Can you work these out from the model? Positions are in its coordinate system, mm. A direction names the side the tool comes from. Coordinates: 2 decimals unless noted, no trailing zeros. Write each loop counter-clockwise with the first axis right and the second up, starting at its lowest first coordinate (ties: lowest second). Pieces come first, ordered by that corner, then holes. Notation, with made-up numbers: M -22.75,-16.75 L 15.25,-16.75 A20 ccw 15.25,-7.75 Z; hole C 70.5,31 d10. An arc over 180 degrees is marked long. Answer as a JSON object with one key per item and string values. Group by question number.
from build123d import *

# Parameters (mm, degrees)
BOSS_EXTRUDE1_DEPTH = 1.4
BOSS_EXTRUDE2_START = -8.5
FRONT_FACE_3_W      = 155.03
FRONT_FACE_3_H      = 88.87
BOSS_EXTRUDE2_DEPTH = 8.5


with BuildPart() as part:
    # Front Face → Boss-Extrude1 (new body)
    with BuildSketch(Plane(origin=(0, 0, 0), x_dir=(1, 0, 0), z_dir=(0, 1, 0))):
        with BuildLine():
            ThreePointArc((0, 120.76), (2.928932188, 127.831067812), (10, 130.76))
            Line((10, 130.76), (202.96, 130.76))
            ThreePointArc((202.96, 130.76), (210.031067812, 127.831067812), (212.96, 120.76))
            Line((212.96, 120.76), (212.96, 10))
            ThreePointArc((212.96, 10), (210.031067812, 2.928932188), (202.96, 0))
            Line((202.96, 0), (10, 0))
            ThreePointArc((10, 0), (2.928932188, 2.928932188), (0, 10))
            Line((0, 10), (0, 120.76))
        make_face()
        with BuildLine():
            Line((10, 16), (10, 114.76))
            ThreePointArc((10, 114.76), (11.757359313, 119.002640687), (16, 120.76))
            Line((16, 120.76), (196.96, 120.76))
            ThreePointArc((196.96, 120.76), (201.202640687, 119.002640687), (202.96, 114.76))
            Line((202.96, 114.76), (202.96, 16))
            ThreePointArc((202.96, 16), (201.202640687, 11.757359313), (196.96, 10))
            Line((196.96, 10), (16, 10))
            ThreePointArc((16, 10), (11.757359313, 11.757359313), (10, 16))
        make_face(mode=Mode.SUBTRACT)
    extrude(amount=BOSS_EXTRUDE1_DEPTH)

    # Front Face_3 → Boss-Extrude2 (add)
    with BuildSketch(Plane(origin=(0, 0, 0), x_dir=(1, 0, 0), z_dir=(0, 1, 0)).offset(BOSS_EXTRUDE2_START)):
        with BuildLine():
            ThreePointArc((0, 10), (2.928932188, 2.928932188), (10, 0))
            Line((10, 0), (202.96, 0))
            ThreePointArc((202.96, 0), (210.031067812, 2.928932188), (212.96, 10))
            Line((212.96, 10), (212.96, 120.76))
            ThreePointArc((212.96, 120.76), (210.031067812, 127.831067812), (202.96, 130.76))
            Line((202.96, 130.76), (10, 130.76))
            ThreePointArc((10, 130.76), (2.928932188, 127.831067812), (0, 120.76))
            Line((0, 120.76), (0, 10))
        make_face()
        with Locations((106.48, 64.38)):
            Rectangle(FRONT_FACE_3_W, FRONT_FACE_3_H, mode=Mode.SUBTRACT)
    extrude(amount=BOSS_EXTRUDE2_DEPTH)


solid = part.part
Q1. Please list where these lines run through material, in increasing order: L1, parallel to Z at x = 165, y = -6.75 (3 decimals); L2, parallel to X at y = -7.5, z = -87 (3 decimals); L3, parallel to Y at x = 11.5, z = -71.5.
Q2. If we section it at C-C on x = 115: List the corners of the cut face in (y, z) for me (3 decimals).
Q3. Will this pin go through, and if not, where does the flat tip stop? pin 1 (1 mm diameter, centred on x = 186.5, z = -21, fed in from +Y).
Q4. On a 3-axis mill with a long thin cutter (end or side, diameter ignored), from which of +Z, -Z, +X, -X, +Y, -Y can I reach the whole of each face in a straight line? I mean faces 1 (the cylindrical face through (201.156, 0.69, -119.049)), 2 (the flat face through (183.995, -4, -64)), 3 (the flat face through (108, -4, -130.76)). Say none if no direction works.
Q5. If we section it at D-D on x = 188: List the corners of the cut face in (y, z) for me.
Q6. We'd pull the mould along X, two halves only. Please class faces 4 (the cylindrical face through (201.249, 0.69, -11.804)), 5 (the cylindrical face through (210.11, -3.62, -127.75)), 6 (the cylindrical face through (3, -3.6, -127.9)): pulls with the +X half, pulls with the -X half, needs draft (parallel to the pull), parting line crosses it, or undercut.
Q7. If we section it at A-A on z = -74.5: List the corners of the cut face in (x, y) for me (3 decimals).
Q8. If we section it at B-B on y = -2.5: List the corners of the cut face in (x, z) for me (3 decimals), and give its area (3 significant figures).
Reply:
{
 "1": {"L1": "-130.76 to -108.815, -19.945 to 0", "L2": "0 to 28.965, 183.995 to 212.96", "L3": "-8.5 to 0"},
 "2": {"outline": "M -8.5,-130.76 L 1.4,-130.76 L 1.4,-120.76 L 0,-120.76 L 0,-108.815 L -8.5,-108.815 Z; M -8.5,-19.945 L 0,-19.945 L 0,-10 L 1.4,-10 L 1.4,0 L -8.5,0 Z"},
 "3": {"pin 1": "y = 0"},
 "4": {"face 1": "+Y", "face 2": "+Y, -Y", "face 3": "-Z, +X, -X, +Y, -Y"},
 "5": {"outline": "M -8.5,-130.76 L 1.4,-130.76 L 1.4,-120.76 L 0,-120.76 L 0,-10 L 1.4,-10 L 1.4,0 L -8.5,0 Z"},
 "6": {"face 4": "undercut", "face 5": "pulls with the +X half", "face 6": "pulls with the -X half"},
 "7": {"outline": "M 0,-8.5 L 28.965,-8.5 L 28.965,0 L 10,0 L 10,1.4 L 0,1.4 Z; M 183.995,-8.5 L 212.96,-8.5 L 212.96,1.4 L 202.96,1.4 L 202.96,0 L 183.995,0 Z"},
 "8": {"outline": "M 0,-120.76 A10 ccw 10,-130.76 L 202.96,-130.76 A10 ccw 212.96,-120.76 L 212.96,-10 A10 ccw 202.96,0 L 10,0 A10 ccw 0,-10 Z; hole M 28.965,-108.815 L 183.995,-108.815 L 183.995,-19.945 L 28.965,-19.945 Z", "area": "14,000 mm^2"}
}
